```python
from build123d import *

# Parameters (mm, degrees)
F0_W           = 39
F0_H           = 40
F1_DEPTH       = 4
F4_DEPTH       = 25
F5_W           = 39
F5_H           = 7.9928017035
F6_DEPTH       = 25
F9_D           = 1.6
F9_CSINK_D     = 3.8
F9_CSINK_ANGLE = 90
F10_DEPTH      = 2
F12_DEPTH      = 0.9
F13_DEPTH      = 2


with BuildPart() as f1:
    # F0 (on Top) → F1 (new body)
    with BuildSketch(Plane.XY):
        Rectangle(F0_W, F0_H)
    extrude(amount=F1_DEPTH)

    # F3 (on face) → F4 (cut)
    with BuildSketch(Plane.XY.offset(4)):
        with BuildLine():
            Line((-16.7006288041, -20), (16.7006288041, -20))
            ThreePointArc((16.7006288041, -20), (0, -11.3886078894), (-16.7006288041, -20))
        make_face()
        with BuildLine():
            ThreePointArc((-16.7006288041, -20), (-6.2404771258, -51.4156774402), (20.5, -31.8886078894))
            ThreePointArc((20.5, -31.8886078894), (19.5270695508, -25.6481307636), (16.7006288041, -20))
            Line((16.7006288041, -20), (-16.7006288041, -20))
        make_face()
    extrude(amount=-F4_DEPTH, mode=Mode.SUBTRACT)

    # F5 (on face) → F6 (cut)
    with BuildSketch(Plane.XY.offset(4)):
        with Locations((0, 16.0035991482)):
            Rectangle(F5_W, F5_H)
    extrude(amount=-F6_DEPTH, mode=Mode.SUBTRACT)

    # F9 (through all)
    with Locations(Plane.XY.offset(4)):
        with Locations((18, 9), (18, -9), (-18, 9), (-18, -9)):
            CounterSinkHole(F9_D / 2, F9_CSINK_D / 2, counter_sink_angle=F9_CSINK_ANGLE)

    # F7 (on face) → F10 (cut)
    with BuildSketch(Plane.XY.offset(4)):
        with BuildLine():
            Line((0.5, 10.6266411021), (-0.5, 10.6266411021))
            Line((-0.5, 10.6266411021), (-0.5, -11.3947063575))
            ThreePointArc((-0.5, -11.3947063575), (0, -11.3886078894), (0.5, -11.3947063575))
            Line((0.5, -11.3947063575), (0.5, 10.6266411021))
        make_face()
        with BuildLine():
            ThreePointArc((-5.2656999319, -12.0764297096), (-3.9629214288, -11.7752975267), (-2.6432830651, -11.5597354505))
            Line((-2.6432830651, -11.5597354505), (-1.522443646, 10.6266411021))
            Line((-1.522443646, 10.6266411021), (-2.021334134, 10.6266411021))
            Line((-2.021334134, 10.6266411021), (-2.4928057101, 10.6266411021))
            Line((-2.4928057101, 10.6266411021), (-2.9997361505, 10.6266411021))
            Line((-2.9997361505, 10.6266411021), (-5.2656999319, -12.0764297096))
        make_face()
        with BuildLine():
            ThreePointArc((-11.0458529252, -14.6190064709), (-9.5659756043, -13.7573610835), (-8.0193476987, -13.0222340331))
            Line((-8.0193476987, -13.0222340331), (-4.491522759, 10.6266411021))
            Line((-4.491522759, 10.6266411021), (-4.9930326641, 10.6266411021))
            Line((-4.9930326641, 10.6266411021), (-5.5073648691, 10.6266411021))
            Line((-5.5073648691, 10.6266411021), (-6.005277995, 10.6266411021))
            Line((-6.005277995, 10.6266411021), (-11.0458529252, -14.6190064709))
        make_face()
        with BuildLine():
            ThreePointArc((-16.7006288041, -20), (-15.6412505167, -18.6371444882), (-14.4709725994, -17.3682445321))
            Line((-14.4709725994, -17.3682445321), (-7.4931742786, 10.6266411021))
            Line((-7.4931742786, 10.6266411021), (-7.993305102, 10.6266411021))
            Line((-7.993305102, 10.6266411021), (-8.507637307, 10.6266411021))
            Line((-8.507637307, 10.6266411021), (-9.0164762619, 10.6266411021))
            Line((-9.0164762619, 10.6266411021), (-18.1983038783, -20))
            Line((-18.1983038783, -20), (-17.6982320845, -20))
            Line((-17.6982320845, -20), (-16.7006288041, -20))
        make_face()
    extrude(amount=-F10_DEPTH, mode=Mode.SUBTRACT)

    # F11 (on face) → F12 (join)
    with BuildSketch(Plane(origin=(0, 0, 0), x_dir=(1, 0, 0), z_dir=(0, 0, -1))):
        with BuildLine():
            Line((1.5, 0), (6.9393398282, 5.4393398282))
            ThreePointArc((6.9393398282, 5.4393398282), (6.6141807012, 5.9259748515), (6.5, 6.5))
            ThreePointArc((6.5, 6.5), (5.9259748515, 6.6141807012), (5.4393398282, 6.9393398282))
            Line((5.4393398282, 6.9393398282), (0, 1.5))
            Line((0, 1.5), (1.5, 0))
        make_face()
        with BuildLine():
            ThreePointArc((6.5, 6.5), (6.6141807012, 5.9259748515), (6.9393398282, 5.4393398282))
            ThreePointArc((6.9393398282, 5.4393398282), (8.5740251485, 5.1141807012), (9.5, 6.5))
            ThreePointArc((9.5, 6.5), (9.0606601718, 7.5606601718), (8, 8))
            ThreePointArc((8, 8), (7.5606601718, 6.9393398282), (6.5, 6.5))
        make_face()
        with BuildLine():
            Line((6.5645856533, -5.0645856533), (1.5, 0))
            Line((1.5, 0), (0, -1.5))
            Line((0, -1.5), (5.4393398282, -6.9393398282))
            ThreePointArc((5.4393398282, -6.9393398282), (6.1413193654, -6.5435151211), (6.9468304687, -6.5680982812))
            ThreePointArc((6.9468304687, -6.5680982812), (6.5462462433, -5.8695943925), (6.5645856533, -5.0645856533))
        make_face()
        Polygon((0, -1.5), (1.5, 0), (0, 1.5), (-1.5, 0), align=None)
        with BuildLine():
            ThreePointArc((5.4393398282, 6.9393398282), (5.9259748515, 6.6141807012), (6.5, 6.5))
            ThreePointArc((6.5, 6.5), (6.9393398282, 7.5606601718), (8, 8))
            ThreePointArc((8, 8), (5.9259748515, 9.3858192988), (5.4393398282, 6.9393398282))
        make_face()
        with BuildLine():
            ThreePointArc((8, 8), (6.9393398282, 7.5606601718), (6.5, 6.5))
            ThreePointArc((6.5, 6.5), (7.5606601718, 6.9393398282), (8, 8))
        make_face()
        with BuildLine():
            Line((-5.4393398282, -6.9393398282), (0, -1.5))
            Line((0, -1.5), (-1.5, 0))
            Line((-1.5, 0), (-6.5645856533, -5.0645856533))
            ThreePointArc((-6.5645856533, -5.0645856533), (-5.7951926461, -5.6064457263), (-5.5, -6.5))
            ThreePointArc((-5.5, -6.5), (-5.5102000145, -6.6746310491), (-5.5406613378, -6.8468871126))
            ThreePointArc((-5.5406613378, -6.8468871126), (-5.4889432763, -6.8919547385), (-5.4393398282, -6.9393398282))
        make_face()
        with BuildLine():
            ThreePointArc((9.5, -5.5), (8.2200891637, -4.0162342638), (6.5645856533, -5.0645856533))
            ThreePointArc((6.5645856533, -5.0645856533), (6.5462462433, -5.8695943925), (6.9468304687, -6.5680982812))
            ThreePointArc((6.9468304687, -6.5680982812), (7.2717436331, -6.7137606114), (7.5531695313, -6.9319017188))
            ThreePointArc((7.5531695313, -6.9319017188), (8.8887503297, -6.7083554326), (9.5, -5.5))
        make_face()
        with BuildLine():
            Line((-1.5, 0), (0, 1.5))
            Line((0, 1.5), (-5.4393398282, 6.9393398282))
            ThreePointArc((-5.4393398282, 6.9393398282), (-5.9259748515, 6.6141807012), (-6.5, 6.5))
            ThreePointArc((-6.5, 6.5), (-6.6141807012, 5.9259748515), (-6.9393398282, 5.4393398282))
            Line((-6.9393398282, 5.4393398282), (-1.5, 0))
        make_face()
        with BuildLine():
            ThreePointArc((-5, -8), (-5.1141807012, -7.4259748515), (-5.4393398282, -6.9393398282))
            Line((-5.4393398282, -6.9393398282), (-5.6464466094, -7.1464466094))
            ThreePointArc((-5.6464466094, -7.1464466094), (-5.9393398282, -7.5606601718), (-6.3535533906, -7.8535533906))
            ThreePointArc((-6.3535533906, -7.8535533906), (-7.185794128, -7.9884490391), (-7.9593386622, -7.6531128874))
            ThreePointArc((-7.9593386622, -7.6531128874), (-6.6746310491, -9.4897999855), (-5, -8))
        make_face()
        with BuildLine():
            Line((-5.6464466094, -7.1464466094), (-5.4393398282, -6.9393398282))
            ThreePointArc((-5.4393398282, -6.9393398282), (-5.4889432763, -6.8919547385), (-5.5406613378, -6.8468871126))
            ThreePointArc((-5.5406613378, -6.8468871126), (-5.585601047, -6.9994753265), (-5.6464466094, -7.1464466094))
        make_face()
        with BuildLine():
            ThreePointArc((6.9468304687, -6.5680982812), (6.1413193654, -6.5435151211), (5.4393398282, -6.9393398282))
            ThreePointArc((5.4393398282, -6.9393398282), (5.9259748515, -9.3858192988), (8, -8))
            ThreePointArc((8, -8), (7.8837908615, -7.421102037), (7.5531695313, -6.9319017188))
            ThreePointArc((7.5531695313, -6.9319017188), (7.2282563669, -6.7862393886), (6.9468304687, -6.5680982812))
        make_face()
        with BuildLine():
            ThreePointArc((7.5531695313, -6.9319017188), (7.2717436331, -6.7137606114), (6.9468304687, -6.5680982812))
            ThreePointArc((6.9468304687, -6.5680982812), (7.2282563669, -6.7862393886), (7.5531695313, -6.9319017188))
        make_face()
        with BuildLine():
            ThreePointArc((-6.5, 6.5), (-5.9259748515, 6.6141807012), (-5.4393398282, 6.9393398282))
            ThreePointArc((-5.4393398282, 6.9393398282), (-5.1141807012, 7.4259748515), (-5, 8))
            ThreePointArc((-5, 8), (-6.5, 9.5), (-8, 8))
            ThreePointArc((-8, 8), (-6.9393398282, 7.5606601718), (-6.5, 6.5))
        make_face()
        with BuildLine():
            Line((-6.3535533906, -7.8535533906), (-5.6464466094, -7.1464466094))
            ThreePointArc((-5.6464466094, -7.1464466094), (-5.585601047, -6.9994753265), (-5.5406613378, -6.8468871126))
            ThreePointArc((-5.5406613378, -6.8468871126), (-6.974341649, -6.5769750529), (-7.9593386622, -7.6531128874))
            ThreePointArc((-7.9593386622, -7.6531128874), (-7.185794128, -7.9884490391), (-6.3535533906, -7.8535533906))
        make_face()
        with BuildLine():
            ThreePointArc((-7.9593386622, -7.6531128874), (-6.974341649, -6.5769750529), (-5.5406613378, -6.8468871126))
            ThreePointArc((-5.5406613378, -6.8468871126), (-5.5102000145, -6.6746310491), (-5.5, -6.5))
            ThreePointArc((-5.5, -6.5), (-5.7951926461, -5.6064457263), (-6.5645856533, -5.0645856533))
            ThreePointArc((-6.5645856533, -5.0645856533), (-8.3205084182, -5.7884822437), (-7.9593386622, -7.6531128874))
        make_face()
        with BuildLine():
            ThreePointArc((-8, 8), (-9.3858192988, 5.9259748515), (-6.9393398282, 5.4393398282))
            ThreePointArc((-6.9393398282, 5.4393398282), (-6.6141807012, 5.9259748515), (-6.5, 6.5))
            ThreePointArc((-6.5, 6.5), (-7.5606601718, 6.9393398282), (-8, 8))
        make_face()
        with BuildLine():
            ThreePointArc((-8, 8), (-7.5606601718, 6.9393398282), (-6.5, 6.5))
            ThreePointArc((-6.5, 6.5), (-6.9393398282, 7.5606601718), (-8, 8))
        make_face()
    extrude(amount=F12_DEPTH)

    # F7 (on face) → F13 (cut)
    with BuildSketch(Plane.XY.offset(4)):
        with BuildLine():
            Line((0.5, 10.6266411021), (-0.5, 10.6266411021))
            Line((-0.5, 10.6266411021), (-0.5, -11.3947063575))
            ThreePointArc((-0.5, -11.3947063575), (0, -11.3886078894), (0.5, -11.3947063575))
            Line((0.5, -11.3947063575), (0.5, 10.6266411021))
        make_face()
        with BuildLine():
            Line((1.522443646, 10.6266411021), (2.6491718308, -11.5605020108))
            ThreePointArc((2.6491718308, -11.5605020108), (3.9661171857, -11.7759274497), (5.2662566492, -12.0765776829))
            Line((5.2662566492, -12.0765776829), (2.9997361505, 10.6266411021))
            Line((2.9997361505, 10.6266411021), (2.498709131, 10.6266411021))
            Line((2.498709131, 10.6266411021), (2.0272377878, 10.6266411021))
            Line((2.0272377878, 10.6266411021), (1.522443646, 10.6266411021))
        make_face()
        with BuildLine():
            Line((4.491522759, 10.6266411021), (8.0269443273, -13.0254648648))
            ThreePointArc((8.0269443273, -13.0254648648), (9.5712306064, -13.7601345759), (11.048909782, -14.620962056))
            Line((11.048909782, -14.620962056), (6.005277995, 10.6266411021))
            Line((6.005277995, 10.6266411021), (5.4984204471, 10.6266411021))
            Line((5.4984204471, 10.6266411021), (4.9972091801, 10.6266411021))
            Line((4.9972091801, 10.6266411021), (4.491522759, 10.6266411021))
        make_face()
        with BuildLine():
            ThreePointArc((-16.7006288041, -20), (-15.6412505167, -18.6371444882), (-14.4709725994, -17.3682445321))
            Line((-14.4709725994, -17.3682445321), (-7.4931742786, 10.6266411021))
            Line((-7.4931742786, 10.6266411021), (-7.993305102, 10.6266411021))
            Line((-7.993305102, 10.6266411021), (-8.507637307, 10.6266411021))
            Line((-8.507637307, 10.6266411021), (-9.0164762619, 10.6266411021))
            Line((-9.0164762619, 10.6266411021), (-18.1983038783, -20))
            Line((-18.1983038783, -20), (-17.6982320845, -20))
            Line((-17.6982320845, -20), (-16.7006288041, -20))
        make_face()
        with BuildLine():
            Line((7.4931742786, 10.6266411021), (14.4761775715, -17.3734336598))
            ThreePointArc((14.4761775715, -17.3734336598), (15.6436257508, -18.6399485848), (16.7006288041, -20))
            Line((16.7006288041, -20), (17.7064798772, -20))
            Line((17.7064798772, -20), (18.2065498084, -20))
            Line((18.2065498084, -20), (9.0164762619, 10.6266411021))
            Line((9.0164762619, 10.6266411021), (8.5177253932, 10.6266411021))
            Line((8.5177253932, 10.6266411021), (7.9971281812, 10.6266411021))
            Line((7.9971281812, 10.6266411021), (7.4931742786, 10.6266411021))
        make_face()
    extrude(amount=-F13_DEPTH, mode=Mode.SUBTRACT)


solid = f1.part
```
Read the model definition and answer for the solid it produces. Units are mm, in the model's axes. A direction names the side the tool comes from. Coordinates: 2 decimals unless noted, no trailing zeros. Order: outer loops, then holes, each group sorted by start corner. A loop starts at its lowest first (then second) coordinate and runs counter-clockwise, first axis right, second up. Notation, with made-up numbers: (-19.5, 87.5) - (35.5, 87.5) arc R9 ccw to (35.5, 101.5) - close; hole circle Ø3 at (37.5, 14.5). An arc over 180 degrees is marked (long way). Answer as a JSON object with one key per item and string values. Group by question number.
Item 1: The mould has two halves that part along Y. Classify faces 4 (the face through (0, 12.007, 2)), 5 (the face through (-18.4, -20, 1.5)), 6 (the face through (-3, -1, 2)): +Y half, -Y half, draft (parallel to the pull), parting line (faces both ways), or undercut.
Item 2: Flat-ended cylindrical pins translate along their axes: P1, Ø1, axis at x = -15, z = 1.5, coming from the -Y side; P2, Ø1.8, axis at x = 18, y = -9, coming from the +Z side; P3, Ø2, axis at x = -18, y = 9, coming from the -Z side. Find the tip coordinate at first contact, or state that the pin passes through.
Item 3: Section D-D (x = 14) is taken. Give the vertices of the cut face in (y, z), plus the area to 3 significant figures.
Item 4: Section A-A (z = 1.4) is taken. Give the vertices of the cut face in (x, y).
Item 5: Section C-C (y = -9) is taken. State how many separate pieces and enclosed holes the cut face has, plus the area to 3 significant figures.
Item 6: A tool of negligible diameter and unlimited length cuts with its end or side. For faces 1 (the face through (-4.117, -0.566, 3.014)), 2 (the face through (4.1, 2.6, -0.4)), 3 (the face through (8, -3, 2)), from which of +Z, -Z, +X, -X, +Y, -Y can it reach the whole face along a straight path? Write none if from no direction.
Item 7: Consider probe 1 along Y at (x, z) = (-18, 1.75); probe 2 along X at (y, z) = (9, 0.75); probe 3 along X at (y, z) = (-14.5, 3.05). Determine where each line is inside the solid, lowest interval first. Write a range as from..to.
Item 8: Section B-B (x = 3.5) is taken. Give the vertices of the cut face in (y, z), plus the area to 3 significant figures.
Results are:
{
 "1": {"face 4": "+Y half", "face 5": "-Y half", "face 6": "undercut"},
 "2": {"P1": "stops at y = -18.47", "P2": "stops at z = 3", "P3": "stops at z = 0"},
 "3": {"outline": "(-16.91, 0) - (12.01, 0) - (12.01, 4) - (-5.98, 4) - (-5.98, 2) - (-15.46, 2) - (-15.46, 4) - (-16.91, 4) - close", "area": "96.7 mm^2"},
 "4": {"outline": "(-19.5, -20) - (-16.7, -20) arc R20.5 cw to (16.7, -20) - (19.5, -20) - (19.5, 12.01) - (-19.5, 12.01) - close; hole circle Ø1.6 at (-18, -9); hole circle Ø1.6 at (-18, 9); hole circle Ø1.6 at (18, -9); hole circle Ø1.6 at (18, 9)"},
 "5": {"separate pieces": "3", "enclosed holes": "0", "area": "113 mm^2"},
 "6": {"face 1": "+Z, -Y", "face 2": "-Z", "face 3": "+Z"},
 "7": {"probe 1": "y = -20..-9.8, -8.2..8.2, 9.8..12.01", "probe 2": "x = -19.5..-18.8, -17.2..17.2, 18.8..19.5", "probe 3": "x = -19.5..-16.55, -13.76..-11.02, 11.02..13.76, 16.56..19.5"},
 "8": {"outline": "(-11.69, 0) - (-5, 0) - (-5, -0.9) - (-2, -0.9) - (-2, 0) - (2, 0) - (2, -0.9) - (5, -0.9) - (5, 0) - (12.01, 0) - (12.01, 4) - (5.62, 4) - (5.62, 2) - (-11.69, 2) - close", "area": "65.6 mm^2"}
}
